CAD build for the part. Positions are in the model's coordinates, mm. Give positions to 0.01 mm unless a question says otherwise; leave off trailing zeros. Write each loop counter-clockwise with the first axis right and the second up, starting at its lowest first coordinate (ties: lowest second). Pieces come first, ordered by that corner, then holes. Notation, with made-up numbers: (51, 64) -> (60, 64) arc R25 ccw to (60, 79) -> close; hole circle Ø6 at (41.25, 1). An arc over 180 degrees is marked (long way). Use one line per item in the form item = value. Start each with the question number.
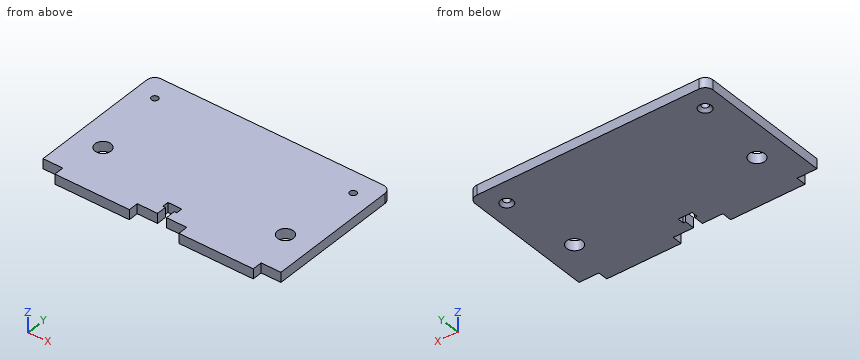
Autodesk Inventor part; units mm, degrees
ref_plane "YZ Plane" through (0, 0, 0) normal (1, 0, 0) x (0, 1, 0)
ref_plane "XZ Plane" through (0, 0, 0) normal (0, 1, 0) x (-1, 0, 0)
ref_plane "XY Plane" through (0, 0, 0) normal (0, 0, 1) x (1, 0, 0)
sketch "Sketch1" plane through (0, 0, 0) normal (0, 0, 1) x (1, 0, 0)
  line L0 (-60, 75) -> (60, 75)
  line L1 (60, 75) -> (60, 5)
  line L2 (60, 5) -> (50, 5)
  line L3 (50, 5) -> (50, 0)
  line L4 (-50, 0) -> (-50, 5)
  line L5 (-50, 5) -> (-60, 5)
  line L6 (-60, 75) -> (-60, 5)
  line L7 (50, 0) -> (12.5, 0)
  line L8 (12.5, 0) -> (12.5, 5)
  line L9 (12.5, 5) -> (-12.5, 5)
  line L10 (-12.5, 5) -> (-12.5, 0)
  line L11 (-12.5, 0) -> (-50, 0)
  point P0 (0, 0)
  point P1 (0, 75)
  point P2 (0, 0)
  point P3 (0, 5)
  dimension "d0" = 5
  dimension "d1" = 100
  dimension "d2" = 120
  dimension "d3" = 70
  dimension "d22" = 5
  dimension "d23" = 25
  dimension "d24" = 5
  dimension "d25" = 10
extrude "Extrusion1" add sketch "Sketch1" along normal blind 5
sketch "Sketch3" plane through (0, 0, 0) normal (0, 0, -1) x (-1, 0, 0)
  line L0 (-50, 63.5) -> (50, 63.5) construction
  line L1 (12.5, 5) -> (-12.5, 5)
  point P0 (0, 0)
  point P1 (0, 63.5)
  dimension "d12" = 100
  dimension "d43" = 58.5
hole "Hole1" at (50, 63.5, 0) at (-50, 63.5, 0) direction (0, 0, 1) diameter 3.4 depth 8 tip angle 118 countersink diameter 6.3 countersink angle 90
fillet "Fillet1" radius 4 2 edges at (60, 75, 2.5) (-60, 75, 2.5)
sketch "Sketch5" plane through (0, 0, 0) normal (0, 0, -1) x (-1, 0, 0)
  line L0 (-2.25, 5) -> (-2.25, 10)
  line L1 (-2.25, 10) -> (-3.5, 10)
  line L2 (-3.5, 10) -> (-3.5, 13.2)
  line L3 (-3.5, 13.2) -> (3.5, 13.2)
  line L4 (3.5, 13.2) -> (3.5, 10)
  line L5 (3.5, 10) -> (2.25, 10)
  line L6 (2.25, 10) -> (2.25, 5)
  line L7 (-12.5, 5) -> (12.5, 5)
  line L8 (-2.25, 5) -> (2.25, 5)
  point P0 (0, 0)
  point P1 (0, 13.2)
  point P2 (0, 5)
  point P3 (0, 5)
  dimension "d26" = 7
  dimension "d27" = 3.2
  dimension "d28" = 5
  dimension "d29" = 4.5
extrude "Extrusion3" cut sketch "Sketch5" against normal blind 5
sketch "Sketch6" plane through (0, 0, 0) normal (0, 0, -1) x (-1, 0, 0)
  line L0 (-60, 71) -> (-60, 5)
  line L1 (56, 75) -> (-56, 75)
  circle A0 centre (-50, 63.5) radius 1.7
  point P0 (0, 0)
  point P1 (-46, 25.5)
  point P2 (46, 25.5)
  dimension "d41" = 4
  dimension "d42" = 38
  dimension "d44" = 92
hole "Hole2" at (46, 25.5, 0) at (-46, 25.5, 0) direction (0, 0, 1) diameter 8 depth 8 tip angle 118
equation "\"d25\" = -0.5 * d1 + 0.5 * d2"
properties part number "LogicHolder" material "Polycarbonate, Clear"
1) Cut at B-B (z = 3.5). Give the cut face in (x, y).
2) Cut at C-C (x = 9.5). Give the cut face in (y, z), and give its area (3 significant figures).
3) Cut at A-A (y = 63.5). Give the cut face in (x, z).
4) Pin check, flat tips, straight feed: pin 1 (2 mm diameter, centred on x = -0.5, z = 1, fed in from -Y); pin 2 (4 mm diameter, centred on x = 50, y = 63.5, fed in from -Z); pin 3 (1.5 mm diameter, centred on x = 56.5, z = 3.5, fed in from -Y). Stop position of each tip, or through.
5) Cut at D-D (y = 25.5). Give the cut face in (x, z), and give its area (3 significant figures).
6) Wall check: line 1 along X through (y, z) = (63.5, 4.2); line 2 along X through (y, z) = (25.5, 2.95); line 3 along X through (y, z) = (6, 3.85). Give the ranges that are in metal, low to high. Write a range as from..to.
Final values:
q1.outline = (-60, 5) -> (-50, 5) -> (-50, 0) -> (-12.5, 0) -> (-12.5, 5) -> (-2.25, 5) -> (-2.25, 10) -> (-3.5, 10) -> (-3.5, 13.2) -> (3.5, 13.2) -> (3.5, 10) -> (2.25, 10) -> (2.25, 5) -> (12.5, 5) -> (12.5, 0) -> (50, 0) -> (50, 5) -> (60, 5) -> (60, 71) arc R4 ccw to (56, 75) -> (-56, 75) arc R4 ccw to (-60, 71) -> close; hole circle Ø3.4 at (-50, 63.5); hole circle Ø8 at (-46, 25.5); hole circle Ø8 at (46, 25.5); hole circle Ø3.4 at (50, 63.5)
q2.outline = (5, 0) -> (75, 0) -> (75, 5) -> (5, 5) -> close
q2.area = 350 mm^2
q3.outline = (-60, 0) -> (-53.15, 0) -> (-51.7, 1.45) -> (-51.7, 5) -> (-60, 5) -> close; (-48.3, 1.45) -> (-46.85, 0) -> (46.85, 0) -> (48.3, 1.45) -> (48.3, 5) -> (-48.3, 5) -> close; (51.7, 1.45) -> (53.15, 0) -> (60, 0) -> (60, 5) -> (51.7, 5) -> close
q4.pin_1 = 13.2
q4.pin_2 = 1.15
q4.pin_3 = 5
q5.outline = (-60, 0) -> (-50, 0) -> (-50, 5) -> (-60, 5) -> close; (-42, 0) -> (42, 0) -> (42, 5) -> (-42, 5) -> close; (50, 0) -> (60, 0) -> (60, 5) -> (50, 5) -> close
q5.area = 520 mm^2
q6.line_1 = -60..-51.7, -48.3..48.3, 51.7..60
q6.line_2 = -60..-50, -42..42, 50..60
q6.line_3 = -60..-2.25, 2.25..60
